Autodesk Inventor part; units mm, degrees
ref_plane "YZ Plane" through (0, 0, 0) normal (1, 0, 0) x (0, 1, 0)
ref_plane "XZ Plane" through (0, 0, 0) normal (0, 1, 0) x (-1, 0, 0)
ref_plane "XY Plane" through (0, 0, 0) normal (0, 0, 1) x (1, 0, 0)
sketch "Sketch1" plane through (0, 0, 0) normal (0, 0, 1) x (1, 0, 0)
  line L0 (-28.8758, -59.7214) -> (-28.8758, 21.7165)
  line L1 (-18.8555, -59.7214) -> (-80.3235, -59.7214)
  line L2 (-57.4508, -59.7214) -> (-57.4508, 50.7628)
  line L3 (-28.8758, 21.7165) -> (27.7449, -35.838)
  line L4 (27.7449, -35.838) -> (27.7449, -59.7214)
  line L5 (-57.4508, 50.7628) -> (-35.9111, 60.559)
  line L6 (-35.9111, 60.559) -> (82.4177, -59.7214)
  line L7 (82.4177, -59.7214) -> (27.7449, -59.7214)
  arc A0 (27.7449, -59.7214) -> (8.6214, -16.3991) centre (-46.0524, -66.4154) ccw
  circle A1 centre (45.7367, -33.5276) radius 2.3241
  circle A2 centre (45.7367, -46.2276) radius 2.3241
  circle A3 centre (26.6867, -27.9714) radius 2.3241
  circle A4 centre (35.7401, -19.0649) radius 2.3241
  circle A5 centre (-35.5854, 44.3824) radius 2.3241
  circle A6 centre (-26.6789, 35.329) radius 2.3241
  point P0 (0, 0)
  dimension "d0" = 90
  dimension "d1" = 90
  dimension "d2" = 4.6482
  dimension "d3" = 4.6482
  dimension "d4" = 4.6482
  dimension "d5" = 4.6482
  dimension "d6" = 4.6482
  dimension "d7" = 4.6482
extrude "Extrusion1" add sketch "Sketch1" along normal blind 15.8877
sketch "Sketch2" plane through (0, 0, 0) normal (0, 0, -1) x (-1, 0, 0)
  line L0 (28.8758, -59.7214) -> (28.8758, 21.7165)
  line L1 (57.4508, -59.7214) -> (28.8758, -59.7214)
  line L2 (57.4508, 50.7628) -> (57.4508, -59.7214)
  line L3 (28.8758, -59.7214) -> (30.4633, -59.7214)
  line L4 (57.4508, -59.7214) -> (55.8633, -59.7214)
  line L5 (30.4633, -59.7214) -> (30.4633, -46.2594)
  line L6 (30.4633, -46.2594) -> (55.8633, -46.2594)
  line L7 (55.8633, -46.2594) -> (55.8633, -59.7214)
  line L8 (28.8758, -59.7214) -> (28.8758, -46.2594)
  line L9 (30.4633, -46.2594) -> (28.8758, -46.2594)
  line L10 (55.8633, -46.2594) -> (57.4508, -46.2594)
  line L11 (57.4508, -59.7214) -> (57.4508, -46.2594)
  point P0 (0, 0)
  dimension "d10" = 1.5875
  dimension "d11" = 1.5875
  dimension "d12" = 13.462
extrude "Extrusion2" cut sketch "Sketch2" against normal blind 4.7752 contours L5 L6 L7 L1
properties part number "Lady Brown Brace"
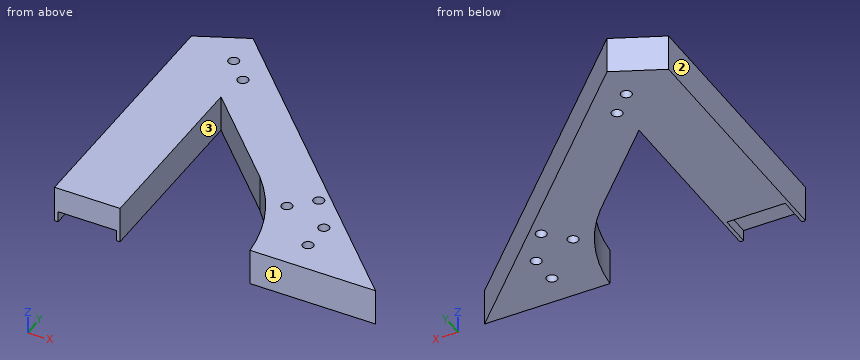
Here's how the part is built. I have some questions about the finished solid (model axes, mm). Face numbers are marked on the shaded views. Coordinates: 2 decimals unless noted, no trailing zeros. Order: outer loops, then holes, each group sorted by start corner. A loop starts at its lowest first (then second) coordinate and runs counter-clockwise, first axis right, second up. Notation, with made-up numbers: (54, 62.25) -> (112, 62.25) arc R23 cw to (112, 78.25) -> close; hole circle Ø2 at (58, 14.5). An arc over 180 degrees is marked (long way). Return JSON: item names as keys, results as strings.
1) Thinking about a two-plate mould opening in X: for the marked faces 1, 2 and 3, which applies, +X half, -X half, draft (parallel to the pull), parting line (faces both ways), or undercut?
Conclusion:
{"face 1": "draft", "face 2": "-X half", "face 3": "undercut"}
2) If we section it at B-B on z = 11: List the corners of the cut face in (x, y) for me, plus the area to 3 significant figures.
Conclusion:
{"outline": "(-57.45, -59.72) -> (-28.88, -59.72) -> (-28.88, 21.72) -> (8.62, -16.4) arc R74.1 cw to (27.74, -59.72) -> (82.42, -59.72) -> (-35.91, 60.56) -> (-57.45, 50.76) -> close; hole circle Ø4.65 at (-35.59, 44.38); hole circle Ø4.65 at (-26.68, 35.33); hole circle Ø4.65 at (26.69, -27.97); hole circle Ø4.65 at (35.74, -19.06); hole circle Ø4.65 at (45.74, -46.23); hole circle Ø4.65 at (45.74, -33.53)", "area": "6,620 mm²"}
3) If I drill on probe 1 along X at (y, z) = (12, 9.25); probe 2 along X at (y, z) = (-53, 7); probe 3 along Y at (x, z) = (-37, 4.25), over which ranges is the centre line in solid material (lowest first)?
Conclusion:
{"probe 1": "x = -57.45 to -28.88, -19.32 to 11.86", "probe 2": "x = -57.45 to -28.88, 26.82 to 75.81", "probe 3": "y = -46.26 to 42.54, 46.23 to 60.06"}
4) I'm going to push flat-ended pins straight in: P1, Ø4, axis at x = -44, y = -53, coming from the -Z side; P2, Ø5, axis at y = 3, z = 7, coming from the +X side; P3, Ø2.5, axis at y = -53, z = 3, coming from the +X side. Where does each tip first touch, or does it pass through?
Conclusion:
{"P1": "stops at z = 4.78", "P2": "stops at x = 23.17", "P3": "stops at x = 77.04"}
5) If we section it at A-A on y = 6: List the corners of the cut face in (x, z) for me.
Conclusion:
{"outline": "(-57.45, 0) -> (-28.88, 0) -> (-28.88, 15.89) -> (-57.45, 15.89) -> close; (-13.41, 0) -> (17.76, 0) -> (17.76, 15.89) -> (-13.41, 15.89) -> close"}
6) If we section it at C-C on y = -23: List the corners of the cut face in (x, z) for me.
Conclusion:
{"outline": "(-57.45, 0) -> (-28.88, 0) -> (-28.88, 15.89) -> (-57.45, 15.89) -> close; (14, 0) -> (46.29, 0) -> (46.29, 15.89) -> (14, 15.89) -> close"}
7) If we section it at D-D on x = -48: List the corners of the cut face in (y, z) for me.
Conclusion:
{"outline": "(-59.72, 4.78) -> (-46.26, 4.78) -> (-46.26, 0) -> (55.06, 0) -> (55.06, 15.89) -> (-59.72, 15.89) -> close"}
